Read the model definition and answer for the solid it produces. Units are mm, in the model's axes. A direction names the side the tool comes from. Round coordinates to 2 decimals unless told otherwise and drop trailing zeros. Loops run counter-clockwise (first coordinate to the right, second up) from the corner with the lowest first, then second, coordinate; pieces in that order, holes last. Notation, with made-up numbers: (60, 87.25) - (70, 87.25) arc R30 ccw to (70, 125.25) - close; hole circle Ø6 at (13, 89.25). An arc over 180 degrees is marked (long way). Answer as CSV lines item,"result".
```python
from build123d import *

# Parameters (mm, degrees)
F0_R     = 20
F1_DEPTH = 25
F2_R     = 10
F3_DEPTH = 40
F4_R     = 5


with BuildPart() as f1:
    # F0 (on Top) → F1 (new body)
    with BuildSketch(Plane.XY):
        Circle(F0_R)
    extrude(amount=-F1_DEPTH)

    # F2 (on Top) → F3 (join)
    with BuildSketch(Plane.XY):
        Circle(F2_R)
    extrude(amount=F3_DEPTH)

    # F4
    f4_edges = [f1.edges().sort_by_distance(p)[0] for p in [
        (-20, 0, -25),
    ]]
    fillet(f4_edges, radius=F4_R)


solid = f1.part
```
1) A cutting plane is placed at C-C, the plane z = 13. Determine the outline of the cut face in (x, y).
Entries:
outline,"circle Ø20 at (0, 0)"
2) A tool of negligible diameter and unlimited length cuts with its end or side. For faces 1 (the face through (-4.336, -19.524, -9.86)), 2 (the face through (-2.17, -9.76, 19.72)), from which of +Z, -Z, +X, -X, +Y, -Y can it reach the whole face along a straight path? Write none if from no direction.
Entries:
face 1,"+Z, -Z"
face 2,"+Z"
3) A cutting plane is placed at A-A, the plane x = 0. Determine the outline of the cut face in (y, z).
Entries:
outline,"(-20, -20) arc R5 ccw to (-15, -25) - (15, -25) arc R5 ccw to (20, -20) - (20, 0) - (10, 0) - (10, 40) - (-10, 40) - (-10, 0) - (-20, 0) - close"
4) Find the intervals of material crossed by line 1 (Z direction, x = -13.5, y = 6.5); line 2 (Y direction, x = 8.5, z = -15); line 3 (Z direction, x = -1, y = 17.5), in increasing order.
Entries:
line 1,"z = -25 to 0"
line 2,"y = -18.1 to 18.1"
line 3,"z = -24.31 to 0"
5) A cutting plane is placed at D-D, the plane z = -13.5. Determine the outline of the cut face in (x, y).
Entries:
outline,"circle Ø40 at (0, 0)"
6) Each of these flat-tipped pins is pushed along its axis until it touches: P1, Ø1, axis at y = 10.5, z = -3.5, coming from the -X side; P2, Ø2, axis at x = -1, z = 21, coming from the -Y side; P3, Ø1, axis at y = -9.5, z = -4.5, coming from the +X side. Where does it stop, or does it pass through?
Entries:
P1,"stops at x = -17.32"
P2,"stops at y = -10"
P3,"stops at x = 17.86"
